```python
from build123d import *

# Parameters (mm, degrees)
SKETCH_1_W                     = 6
SKETCH_1_H                     = 62.4
EXTRUDE_1_DEPTH                = 56.4
SKETCH_3_W                     = 56.4
SKETCH_3_H                     = 6
EXTRUDE_3_DEPTH                = 15
HOLE_WIZARD_M5_1_D             = 4.2
HOLE_WIZARD_M5_1_DEPTH         = 12.4
HOLE_WIZARD_M5_1_TIP           = 1.2618073
SKETCH_6_R                     = 20
CUT_EXTRUDE_1_DEPTH            = 15
SKETCH_7_W                     = 21
SKETCH_7_H                     = 56.4
EXTRUDE_4_DEPTH                = 8
SKETCH_8_W                     = 15
SKETCH_8_H                     = 56.4
CUT_EXTRUDE_2_DEPTH            = 5
HOLE_WIZARD_M5_1_2_D           = 5.5
HOLE_WIZARD_M5_1_2_DEPTH       = 12.4
HOLE_WIZARD_M5_1_2_CBORE_D     = 10
HOLE_WIZARD_M5_1_2_CBORE_DEPTH = 5.4
HOLE_WIZARD_M5_1_2_TIP         = 1.652366702
SKETCH_11_W                    = 10
SKETCH_11_H                    = 30
CUT_EXTRUDE_3_DEPTH            = 5.4
SKETCH_12_W                    = 5.5
SKETCH_12_H                    = 30
CUT_EXTRUDE_4_DEPTH            = 10


with BuildPart() as part:
    # 草图1 → 凸台-拉伸1 (new body)
    with BuildSketch(Plane.XY):
        with Locations((3, 31.2)):
            Rectangle(SKETCH_1_W, SKETCH_1_H)
    extrude(amount=EXTRUDE_1_DEPTH)

    # 草图3 → 凸台-拉伸3 (add)
    with BuildSketch(Plane.ZY):
        with Locations((28.2, 3)):
            Rectangle(SKETCH_3_W, SKETCH_3_H)
    extrude(amount=EXTRUDE_3_DEPTH)

    # Hole Wizard M5 _1
    with Locations(Plane(origin=(6, 0, 0), x_dir=(0, 0, -1), z_dir=(1, 0, 0))):
        with Locations((-51.785, 57.785), (-4.615, 57.785), (-4.615, 10.615), (-51.785, 10.615)):
            Hole(HOLE_WIZARD_M5_1_D / 2, depth=HOLE_WIZARD_M5_1_DEPTH)
            with Locations((0, 0, -(HOLE_WIZARD_M5_1_DEPTH + HOLE_WIZARD_M5_1_TIP / 2))):  # 118° drill point
                Cone(0, HOLE_WIZARD_M5_1_D / 2, HOLE_WIZARD_M5_1_TIP, mode=Mode.SUBTRACT)

    # 草图6 → 切除-拉伸1 (cut)
    with BuildSketch(Plane(origin=(6, 0, 0), x_dir=(0, 0, -1), z_dir=(1, 0, 0))):
        with Locations((-28.2, 34.2)):
            Circle(SKETCH_6_R)
    extrude(amount=-CUT_EXTRUDE_1_DEPTH, mode=Mode.SUBTRACT)

    # 草图7 → 凸台-拉伸4 (add)
    with BuildSketch(Plane.XZ):
        with Locations((-4.5, 28.2)):
            Rectangle(SKETCH_7_W, SKETCH_7_H)
    extrude(amount=EXTRUDE_4_DEPTH)

    # 草图8 → 切除-拉伸2 (cut)
    with BuildSketch(Plane(origin=(0, 6, 0), x_dir=(1, 0, 0), z_dir=(0, 1, 0))):
        with Locations((-7.5, -28.2)):
            Rectangle(SKETCH_8_W, SKETCH_8_H)
    extrude(amount=-CUT_EXTRUDE_2_DEPTH, mode=Mode.SUBTRACT)

    # Hole Wizard M5 _1 2
    with Locations(Plane(origin=(0, 1, 0), x_dir=(1, 0, 0), z_dir=(0, 1, 0))):
        with Locations((-7.5, -13.2), (-7.5, -43.2)):
            CounterBoreHole(HOLE_WIZARD_M5_1_2_D / 2, HOLE_WIZARD_M5_1_2_CBORE_D / 2, HOLE_WIZARD_M5_1_2_CBORE_DEPTH, depth=HOLE_WIZARD_M5_1_2_DEPTH)
            with Locations((0, 0, -(HOLE_WIZARD_M5_1_2_DEPTH + HOLE_WIZARD_M5_1_2_TIP / 2))):  # 118° drill point
                Cone(0, HOLE_WIZARD_M5_1_2_D / 2, HOLE_WIZARD_M5_1_2_TIP, mode=Mode.SUBTRACT)

    # 草图11 → 切除-拉伸3 (cut)
    with BuildSketch(Plane(origin=(0, 1, 0), x_dir=(1, 0, 0), z_dir=(0, 1, 0))):
        with Locations((-7.5, -28.2)):
            Rectangle(SKETCH_11_W, SKETCH_11_H)
    extrude(amount=-CUT_EXTRUDE_3_DEPTH, mode=Mode.SUBTRACT)

    # 草图12 → 切除-拉伸4 (cut)
    with BuildSketch(Plane(origin=(0, -4.4, 0), x_dir=(1, 0, 0), z_dir=(0, 1, 0))):
        with Locations((-7.5, -28.2)):
            Rectangle(SKETCH_12_W, SKETCH_12_H)
    extrude(amount=-CUT_EXTRUDE_4_DEPTH, mode=Mode.SUBTRACT)


solid = part.part
```
Input: part model. Units: mm. Frame: model coordinates. A direction names the side the tool comes from. Coordinates: 2 decimals unless noted, no trailing zeros. Loops run counter-clockwise (first coordinate to the right, second up) from the corner with the lowest first, then second, coordinate; pieces in that order, holes last.
Q1. Section C-C, the plane z = 28.2. Return the cut outline in (x, y).
Results are:
outline: (-15, -8) - (-10.25, -8) - (-10.25, -4.4) - (-12.5, -4.4) - (-12.5, 1) - (-15, 1) - close; (-4.75, -8) - (6, -8) - (6, 14.2) - (0, 14.2) - (0, 1) - (-2.5, 1) - (-2.5, -4.4) - (-4.75, -4.4) - close; (0, 54.2) - (6, 54.2) - (6, 62.4) - (0, 62.4) - close
Q2. Section A-A, the plane y = -2. Return the cut outline in (x, z).
Results are:
outline: (-15, 0) - (6, 0) - (6, 56.4) - (-15, 56.4) - close; hole (-12.5, 13.2) arc R5 ccw to (-2.5, 13.2) - (-2.5, 43.2) arc R5 ccw to (-12.5, 43.2) - close
Q3. Set-up query: faces 5 (the cylindrical face through (2.958, 12.697, 4.342)), 6 (the flat face through (-13, 1, 28)), 7 (the flat face through (-11, -4.4, 28)), 8 (the cylindrical face through (-7.44, -6.23, 45.95)). Return all of +Z, -Z, +X, -X, +Y, -Y with unobstructed straight access to the full face (end or side cutting, diameter ignored); none if empty.
Results are:
face 5: +X, -X
face 6: +Z, -Z, -X, +Y
face 7: +Y
face 8: +Y, -Y
Q4. Mould query, pull axis X, two halves, no side actions, for faces 1 (the flat face through (-4.75, -6, 28)), 2 (the flat face through (0, 18, 41)), 3 (the cylindrical face through (2.958, 10.707, 49.687)), 4 (the flat face through (-10.25, -6, 28)). Classes: +X half, -X half, draft (parallel to the pull), parting line (faces both ways), or undercut.
Results are:
face 1: undercut
face 2: -X half
face 3: draft
face 4: undercut
Q5. Line query: line 1 along Y through (x, z) = (0.5, 4); line 2 along Y through (x, z) = (3.3, 28.2); line 3 along X through (y, z) = (19.5, 53.5). Output: solid intervals per line, ascending.
Results are:
line 1: y = -8 to 8.61, 12.62 to 55.78, 59.79 to 62.4
line 2: y = -8 to 14.2, 54.2 to 62.4
line 3: x = 0 to 6
Q6. Section B-B, the plane x = -7.5. Return the cut outline in (y, z).
Results are:
outline: (-8, 0) - (1, 0) - (1, 8.2) - (-4.4, 8.2) - (-4.4, 10.45) - (-8, 10.45) - close; (-8, 45.95) - (-4.4, 45.95) - (-4.4, 48.2) - (1, 48.2) - (1, 56.4) - (-8, 56.4) - close
Q7. Contact query for flat-ended pins moving along their axis: pin 1 (8 mm diameter, centred on x = -9, z = 34, fed in from +Y); pin 2 (6.5 mm diameter, centred on y = 57.785, z = 4.615, fed in from -X). Output: stop coordinate, or through.
Results are:
pin 1: stops at y = 1
pin 2: stops at x = 0
Q8. Section D-D, the plane y = 34.2. Return the cut outline in (x, z), and give its area (3 significant figures).
Results are:
outline: (0, 0) - (6, 0) - (6, 8.2) - (0, 8.2) - close; (0, 48.2) - (6, 48.2) - (6, 56.4) - (0, 56.4) - close
area: 98.4 mm2
